Input: part model. Units: mm. Frame: model coordinates. Coordinates: 2 decimals unless noted, no trailing zeros. Order: outer loops, then holes, each group sorted by start corner. A loop starts at its lowest first (then second) coordinate and runs counter-clockwise, first axis right, second up. Notation, with made-up numbers: (46, -9.5) - (83, -9.5) arc R24 ccw to (83, 28.5) - close; hole circle Ø3 at (51, 51.5). An arc over 180 degrees is marked (long way). Answer as CSV lines item,"result". Start each with the question number.
Item 1: First-contact query: pin 1 (23 mm diameter, centred on x = -17, z = 0, fed in from +Y); pin 2 (4.5 mm diameter, centred on x = -45, z = -17.5, fed in from -Y); pin 3 (4.5 mm diameter, centred on x = -44.5, z = 19, fed in from +Y). Flat tips, straight axial feed; report the tip coordinate or a pass-through.
Item 2: Section D-D (z = 17.5). Output: boundary loops of the cut face in (x, y), and give its area (3 significant figures).
Item 3: Section A-A (z = 0). Output: boundary loops of the cut face in (x, y).
Item 4: Material intervals for line 1 along Z through (x, y) = (45, 3.9); line 2 along Z through (x, y) = (45, 1.25); line 3 along X through (y, z) = (5.6, -17.5), sorted ascending.
Item 5: Section B-B (x = -17.5). Output: boundary loops of the cut face in (y, z), and give its area (3 significant figures).
Item 6: Section C-C (y = 6). Output: boundary loops of the cut face in (x, z).
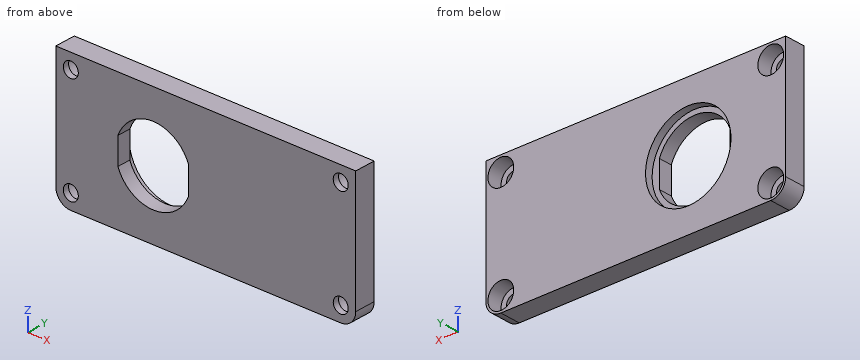
Autodesk Inventor part; units mm, degrees
ref_plane "YZ Plane" through (0, 0, 0) normal (1, 0, 0) x (0, 1, 0)
ref_plane "XZ Plane" through (0, 0, 0) normal (0, 1, 0) x (-1, 0, 0)
ref_plane "XY Plane" through (0, 0, 0) normal (0, 0, 1) x (1, 0, 0)
sketch "Body Outline" plane through (0, 0, 0) normal (0, 1, 0) x (-1, 0, 0)
  line L0 (50, -22.5) -> (-50, -22.5)
  line L1 (-50, -22.5) -> (-50, 22.5)
  line L2 (-50, 22.5) -> (50, 22.5)
  line L3 (50, 22.5) -> (50, -22.5)
  point P0 (0, 0)
  dimension "d0" = 45
  dimension "d1" = 22.5
  dimension "d2" = 100
  dimension "d3" = 50
extrude "Body" add sketch "Body Outline" along normal blind 7
sketch "Connector Hole Cross Section" plane through (0, 7, 0) normal (0, 1, 0) x (1, 0, 0)
  line L0 (-5.7, 4.4181) -> (-5.7, -4.4181)
  line L1 (-29.3, -4.4181) -> (-29.3, 4.4181)
  arc A0 (-5.7, 4.4181) -> (-29.3, 4.4181) centre (-17.5, 0) ccw
  arc A1 (-29.3, -4.4181) -> (-5.7, -4.4181) centre (-17.5, 0) ccw
  line L2 (50, 22.5) -> (-50, 22.5)
  line L3 (-50, 22.5) -> (-50, -22.5)
  point P0 (0, 0)
  dimension "d6" = 11.8
  dimension "d7" = 23.6
  dimension "d8" = 12.6
  dimension "d9" = 12.6
  dimension "d10" = 22.5
  dimension "d12" = 32.5
extrude "Connector Hole" cut sketch "Connector Hole Cross Section" along normal through all both and the other way through all
sketch "Connector Face Hole Cross Section" plane through (0, 7, 0) normal (0, 1, 0) x (1, 0, 0)
  circle A0 centre (-17.5, 0) radius 14.25
  line L0 (50, 22.5) -> (-50, 22.5)
  line L1 (-50, 22.5) -> (-50, -22.5)
  point P0 (0, 0)
  dimension "d15" = 22.5
  dimension "d16" = 32.5
  dimension "d17" = 28.5
extrude "Connector Face Hole" cut sketch "Connector Face Hole Cross Section" against normal blind 2.5
fillet "Body Fillet" radius 5 2 edges at (-50, 3.5, -22.5) (50, 3.5, -22.5)
sketch "Lid Fastening Hole Pattern" plane through (0, 7, 0) normal (0, 1, 0) x (1, 0, 0)
  line L0 (-50, 17.5) -> (-50, -22.5)
  line L1 (45, 22.5) -> (-45, 22.5)
  point P0 (0, 0)
  point P1 (-45, 17.5)
  point P2 (45, 17.5)
  point P3 (-45, -17.5)
  point P4 (45, -17.5)
  dimension "d85" = 5
  dimension "d86" = 5
  dimension "d89" = 90
  dimension "d92" = 35
hole "Lid Fastening Holes" at (-45, 7, -17.5) at (45, 7, -17.5) at (-45, 7, 17.5) at (45, 7, 17.5) direction (0, -1, 0) diameter 5 end through all counterbore diameter 8.6 counterbore depth 5
equation "\"d6\" = 0.5 * d7"
equation "\"d9\" = d8"
equation "\"d10\" = 0.5 * d0"
equation "\"d15\" = 0.5 * d0"
properties part number "Connector Lid" material "Aluminum 6061"
Determined:
1,pin 1,"stops at y = 4.5"
1,pin 2,"passes through"
1,pin 3,"stops at y = 2"
2,outline,"(-50, 0) - (-47.5, 0) - (-47.5, 2) - (-49.3, 2) - (-49.3, 7) - (-50, 7) - close; (-42.5, 0) - (42.5, 0) - (42.5, 2) - (40.7, 2) - (40.7, 7) - (-40.7, 7) - (-40.7, 2) - (-42.5, 2) - close; (47.5, 0) - (50, 0) - (50, 7) - (49.3, 7) - (49.3, 2) - (47.5, 2) - close"
2,area,"594 mm^2"
3,outline,"(-50, 0) - (-29.3, 0) - (-29.3, 4.5) - (-31.75, 4.5) - (-31.75, 7) - (-50, 7) - close; (-5.7, 0) - (50, 0) - (50, 7) - (-3.25, 7) - (-3.25, 4.5) - (-5.7, 4.5) - close"
4,line 1,"z = -22.5 to -21.8, -13.2 to 13.2, 21.8 to 22.5"
4,line 2,"z = -22.5 to -20, -15 to 15, 20 to 22.5"
4,line 3,"x = -50 to -49.3, -40.7 to 40.7, 49.3 to 50"
5,outline,"(0, -22.5) - (7, -22.5) - (7, -14.25) - (4.5, -14.25) - (4.5, -12.6) - (0, -12.6) - close; (0, 12.6) - (4.5, 12.6) - (4.5, 14.25) - (7, 14.25) - (7, 22.5) - (0, 22.5) - close"
5,area,"130 mm^2"
6,outline,"(-50, -17.5) arc R5 ccw to (-45, -22.5) - (45, -22.5) arc R5 ccw to (50, -17.5) - (50, 22.5) - (-50, 22.5) - close; hole circle Ø8.6 at (-45, -17.5); hole circle Ø8.6 at (-45, 17.5); hole circle Ø28.5 at (-17.5, 0); hole circle Ø8.6 at (45, -17.5); hole circle Ø8.6 at (45, 17.5)"
